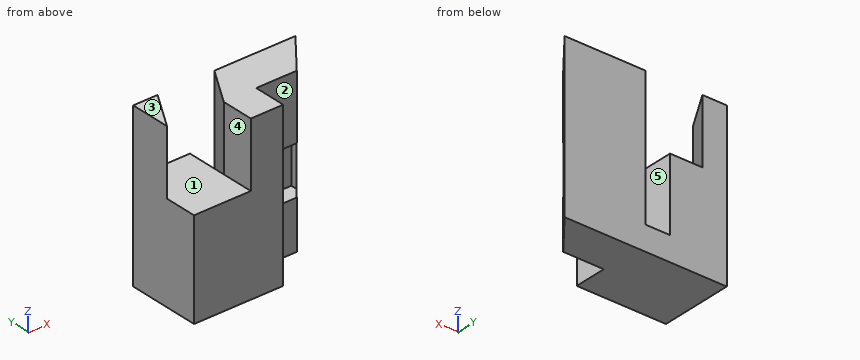
from build123d import *

# Parameters (mm, degrees)
F0_W      = 100
F0_H      = 100
F1_DEPTH  = 45
F2_W      = 45
F2_H      = 100
F3_DEPTH  = 20
F4_W      = 35
F4_H      = 45
F5_DEPTH  = 40
F7_DEPTH  = 40
F10_DEPTH = 100.001
F8_W      = 30
F8_H      = 30
F11_DEPTH = 10
F13_DEPTH = 85


with BuildPart() as f1:
    # F0 (on Front) → F1 (new body)
    with BuildSketch(Plane.XZ):
        with Locations((50, 50)):
            Rectangle(F0_W, F0_H)
    extrude(amount=F1_DEPTH)

    # F2 (on face) → F3 (cut)
    with BuildSketch(Plane.XZ.offset(45)):
        with Locations((77.5, 50)):
            Rectangle(F2_W, F2_H)
    extrude(amount=-F3_DEPTH, mode=Mode.SUBTRACT)

    # F4 (on face) → F5 (cut)
    with BuildSketch(Plane.XY.offset(100)):
        with Locations((17.5, -22.5)):
            Rectangle(F4_W, F4_H)
    extrude(amount=-F5_DEPTH, mode=Mode.SUBTRACT)

    # F6 (on face) → F7 (join)
    with BuildSketch(Plane.XY.offset(60)):
        Polygon((15, 0), (0, 0), (0, -25), align=None)
    extrude(amount=F7_DEPTH)

    # F9 (on face) → F10 (cut, through all)
    with BuildSketch(Plane.XY.offset(100)):
        Polygon((100, -25), (100, 0), (80, -25), align=None)
    extrude(amount=-F10_DEPTH, mode=Mode.SUBTRACT)

    # F8 (on face) → F11 (cut)
    with BuildSketch(Plane.XZ.offset(25)):
        with Locations((70, 45)):
            Rectangle(F8_W, F8_H)
    extrude(amount=-F11_DEPTH, mode=Mode.SUBTRACT)

    # F12 (on face) → F13 (cut)
    with BuildSketch(Plane.XY.offset(100)):
        Polygon((50, 0), (35, 0), (35, -25), align=None)
    extrude(amount=-F13_DEPTH, mode=Mode.SUBTRACT)


solid = f1.part
Build history of the part. All positions in model axes, mm. Face numbers are marked on the shaded views. A direction names the side the tool comes from. Coordinates: 2 decimals unless noted, no trailing zeros. Write each loop counter-clockwise with the first axis right and the second up, starting at its lowest first coordinate (ties: lowest second). Pieces come first, ordered by that corner, then holes. Notation, with made-up numbers: (-22, 57) -> (-12, 57) arc R23 cw to (-12, 78) -> close; hole circle Ø2 at (86.5, 9.25). An arc over 180 degrees is marked (long way). Use CSV: the item, a comma, the result in double quotes. Start each with the question number.
Q1. Cut at A-A, the plane y = -6. List the corners of the cut face in (x, z), then the cut area to 3 significant figures.
Q2. Cut at C-C, the plane y = -17.5. List the corners of the cut face in (x, z), then the cut area to 3 significant figures.
Q3. Drill centre lines: probe 1 along Z at (x, y) = (57.5, -18); probe 2 along X at (y, z) = (-28, 35.5); probe 3 along Y at (x, z) = (78, 69). Where is each one in solid material? Low to high.
Q4. Flat gauge pins, fed straight in: pin 1 Ø3 at (x, z) = (48.5, 15.5) entering from +Y; pin 2 Ø17.5 at (x, y) = (18, -23) entering from +Z; pin 3 Ø3 at (y, z) = (-7, 89) entering from +X; pin 4 Ø1.5 at (y, z) = (-28.5, 10.5) entering from +X. Where does each tip first touch, or does it go through?
Q5. Cut at D-D, the plane x = 60. List the corners of the cut face in (y, z).
Q6. Cut at B-B, the plane z = 37. List the corners of the cut face in (x, y).
Q7. 3-axis set-ups, long thin cutter, end or side, ignore diameter. For the marked faces 1, 2, 3, 4 and 5: which of +Z, -Z, +X, -X, +Y, -Y reach the whole face in a straight line?
Checked values:
1,outline,"(0, 0) -> (95.2, 0) -> (95.2, 100) -> (46.4, 100) -> (46.4, 15) -> (35, 15) -> (35, 60) -> (11.4, 60) -> (11.4, 100) -> (0, 100) -> close"
1,area,"7,610 mm²"
2,outline,"(0, 0) -> (86, 0) -> (86, 100) -> (39.5, 100) -> (39.5, 15) -> (35, 15) -> (35, 60) -> (4.5, 60) -> (4.5, 100) -> (0, 100) -> close; hole (55, 30) -> (85, 30) -> (85, 60) -> (55, 60) -> close"
2,area,"6,100 mm²"
3,probe 1,"z = 0 to 30, 60 to 100"
3,probe 2,"x = 0 to 55"
3,probe 3,"y = -25 to 0"
4,pin 1,"stops at y = 0"
4,pin 2,"stops at z = 60"
4,pin 3,"stops at x = 95.6"
4,pin 4,"stops at x = 55"
5,outline,"(-25, 0) -> (0, 0) -> (0, 100) -> (-25, 100) -> (-25, 60) -> (-15, 60) -> (-15, 30) -> (-25, 30) -> close"
6,outline,"(0, -45) -> (55, -45) -> (55, -15) -> (85, -15) -> (85, -18.75) -> (100, 0) -> (50, 0) -> (35, -25) -> (35, 0) -> (0, 0) -> close"
7,face 1,"+Z, -Y"
7,face 2,"+Z, -Z, +X, -Y"
7,face 3,"+Z, +X, -X, +Y, -Y"
7,face 4,"+Z, -X, +Y, -Y"
7,face 5,"+Z, +Y"
